Geometry check sheet. Reference: the model listing, model coordinates, mm. A direction names the side the tool comes from. Coordinates: 2 decimals unless noted, no trailing zeros. Loops run counter-clockwise (first coordinate to the right, second up) from the corner with the lowest first, then second, coordinate; pieces in that order, holes last. Notation, with made-up numbers: M 52.5,19.5 L 86.5,19.5 A14 ccw 86.5,29.5 Z; hole C -32.75,15.25 d7. An arc over 180 degrees is marked long. Use CSV: the item, a comma, the result in double quotes.
```python
from build123d import *

# Parameters (mm, degrees)
SKICA1_R                 = 50
P_IDAT_VYSUNUT_M1_DEPTH  = 60
SKICA2_R                 = 10
ROTOVAT1_ANGLE           = 90
SKICA3_W                 = 85
SKICA3_H                 = 60
P_IDAT_VYSUNUT_M2_DEPTH  = 100
SKICA4_W                 = 26.634802258
SKICA4_H                 = 52.894466455
ODEBRAT_VYSUNUT_M2_DEPTH = 100
SKICA5_R                 = 7.5
ODEBRAT_VYSUNUT_M3_DEPTH = 100


with BuildPart() as part:
    # Skica1 → Přidat vysunutím1 (new body)
    with BuildSketch(Plane.XY):
        Circle(SKICA1_R)
    extrude(amount=P_IDAT_VYSUNUT_M1_DEPTH)

    # Skica2 → Rotovat1 (revolve)
    with BuildSketch(Plane(origin=(0, 0, 0), x_dir=(-1, 0, 0), z_dir=(0, 0, -1))):
        with Locations((20, -15)):
            Circle(SKICA2_R)
        with Locations((-20, 15)):
            Circle(SKICA2_R)
    revolve(axis=Axis((-92.809652782, 70, 0), (1, 0, 0)), revolution_arc=ROTOVAT1_ANGLE)

    # Skica3 → Přidat vysunutím2 (add)
    with BuildSketch(Plane(origin=(0, 70, 0), x_dir=(1, 0, 0), z_dir=(0, 1, 0))):
        with Locations((-2.5, 70)):
            Rectangle(SKICA3_W, SKICA3_H)
    extrude(amount=P_IDAT_VYSUNUT_M2_DEPTH)

    # Skica4 → Odebrat vysunutím2 (cut)
    with BuildSketch(Plane.ZY.offset(45)):
        with Locations((-91.276231393, 147.219598942)):
            Rectangle(SKICA4_W, SKICA4_H)
    extrude(amount=-ODEBRAT_VYSUNUT_M2_DEPTH, mode=Mode.SUBTRACT)

    # Skica5 → Odebrat vysunutím3 (cut)
    with BuildSketch(Plane.XY.offset(-40)):
        with Locations((20, 90)):
            Circle(SKICA5_R)
        with Locations((-25, 90)):
            Circle(SKICA5_R)
    extrude(amount=-ODEBRAT_VYSUNUT_M3_DEPTH, mode=Mode.SUBTRACT)


solid = part.part
```
1. Set-up check for faces 1 (the flat face through (-3, 145, -77.959)), 2 (the flat face through (-3, 119, -40)), 3 (the flat face through (-1, 1, 0)): record each of +Z, -Z, +X, -X, +Y, -Y from which the full face is reachable in a straight line by a thin tool's end or side.
The answers:
face 1,"-Z, +X, -X, +Y"
face 2,"+Z, +X, -X, +Y"
face 3,"none"
2. Section check A-A, the plane y = 90. Record the cut outline in (x, z), plus the area to 3 significant figures.
The answers:
outline,"M -45,-100 L -32.5,-100 L -32.5,-40 L -45,-40 Z; M -17.5,-100 L 12.5,-100 L 12.5,-40 L -17.5,-40 Z; M 27.5,-100 L 40,-100 L 40,-40 L 27.5,-40 Z"
area,"3,300 mm^2"
3. Section check D-D, the plane y = 151.5. Record the cut outline in (x, z), plus the area to 3 significant figures.
The answers:
outline,"M -45,-77.96 L 40,-77.96 L 40,-40 L -45,-40 Z"
area,"3,230 mm^2"
4. Gauge pin test, flat ends, axial feed: P1, Ø24, axis at x = -9, z = -92.5, coming from the +Y side; P2, Ø1.5, axis at y = 64.5, z = -57, coming from the -X side; P3, Ø12, axis at x = 37, y = 116, coming from the +Z side. Record the tip position at first contact, or that the pin passes through.
The answers:
P1,"y = 120.77"
P2,"x = 10.12"
P3,"z = -40"
5. Thickness scan on line 1 (Y direction, x = 20, z = -83); line 2 (Y direction, x = 33.5, z = -87.5); line 3 (Z direction, x = 29, y = 111.5). Record the ranges inside material, lowest first. Write a range as [from, to].
The answers:
line 1,"[70, 82.5], [97.5, 120.77]"
line 2,"[70, 120.77]"
line 3,"[-100, -40]"
6. Section check B-B, the plane x = 37.5. Record the cut outline in (y, z), plus the area to 3 significant figures.
The answers:
outline,"M -33.07,0 L 33.07,0 L 33.07,60 L -33.07,60 Z; M 70,-100 L 120.77,-100 L 120.77,-77.96 L 170,-77.96 L 170,-40 L 70,-40 Z"
area,"8,880 mm^2"
7. Section check C-C, the plane z = 16.5. Record the cut outline in (x, y).
The answers:
outline,"C 0,0 d100"
8. Release check for a two-part mould opening along X. For faces 4 (the flat face through (-45, 119, -63)), 5 (the flat face through (-3, 170, -59)), 6 (the cylindrical face through (18.37, 82.68, -69.58)) record: +X half, -X half, draft (parallel to the pull), parting line (faces both ways), or undercut.
The answers:
face 4,"-X half"
face 5,"draft"
face 6,"undercut"
